Autodesk Inventor part; units mm, degrees
ref_plane "YZ Plane" through (0, 0, 0) normal (1, 0, 0) x (0, 1, 0)
ref_plane "XZ Plane" through (0, 0, 0) normal (0, 1, 0) x (-1, 0, 0)
ref_plane "XY Plane" through (0, 0, 0) normal (0, 0, 1) x (1, 0, 0)
sketch "Sketch1" plane through (0, 0, 0) normal (0, 0, 1) x (1, 0, 0)
  circle A0 centre (0, 0) radius 11.25
  circle A1 centre (0, 0) radius 12.2
  dimension "d0" = 22.5
  dimension "d1" = 24.4
extrude "Extrusion1" add sketch "Sketch1" along normal blind 6.5
sketch "Sketch2" plane through (0, 0, 0) normal (0, 0, 1) x (1, 0, 0)
  circle A0 centre (0, 0) radius 11.25
  dimension "d4" = 22.5
extrude "Extrusion2" add sketch "Sketch2" along normal blind 1
sketch "Sketch3" plane through (0, 0, 1) normal (0, 0, 1) x (1, 0, 0)
  circle A0 centre (0, 0) radius 9
  dimension "d7" = 18
extrude "Extrusion3" cut sketch "Sketch3" against normal blind 1
properties part number "HubTest22mm"
Geometry check sheet. Reference: the model listing, model coordinates, mm. A direction names the side the tool comes from. Give positions to 0.01 mm unless a question says otherwise; leave off trailing zeros. Order: outer loops, then holes, each group sorted by start corner. A loop starts at its lowest first (then second) coordinate and runs counter-clockwise, first axis right, second up.
1. Release check for a two-part mould opening along X. For faces 3 (the face through (4, -11, 6.5)), 4 (the face through (-5, 8, 1)), 5 (the face through (-12.19, -0.54, 3.2)) record: pulls with the +X half, pulls with the -X half, needs draft (parallel to the pull), parting line crosses it, or undercut.
2. Gauge pin test, flat ends, axial feed: pin 1 Ø1 at (x, z) = (-4, 5.5) entering from -Y; pin 2 Ø2 at (x, z) = (6, 4.5) entering from +Y. Record the tip position at first contact, or that the pin passes through.
3. Section check C-C, the plane z = 5.25. Enter the section's corners in (x, y), and give its area (3 significant figures).
4. Access from +Z, -Z, +X, -X, +Y, -Y to the whole of each face (thin tool, end or side, straight path). Record for faces 1 (the face through (-1.172, 8.923, 0.507)), 2 (the face through (5.19, 9.98, 3.71)).
5. Section check A-A, the plane y = 0. Enter the section's corners in (x, z).
6. Thickness scan on L1, parallel to Y at x = 0, z = 0.4; L2, parallel to Y at x = 0, z = 3; L3, parallel to X at y = -7.75, z = 4. Record the ranges inside material, lowest first.
Values follow:
1. face 3: needs draft
1. face 4: undercut
1. face 5: parting line crosses it
2. pin 1: stops at y = -11.69
2. pin 2: stops at y = 11.13
3. outline: circle Ø24.4 at (0, 0); hole circle Ø22.5 at (0, 0)
3. area: 70.0 mm2
4. face 1: +Z, -Z
4. face 2: +Z
5. outline: (-12.2, 0) - (-9, 0) - (-9, 1) - (-11.25, 1) - (-11.25, 6.5) - (-12.2, 6.5) - close; (9, 0) - (12.2, 0) - (12.2, 6.5) - (11.25, 6.5) - (11.25, 1) - (9, 1) - close
6. L1: y = -12.2 to -9, 9 to 12.2
6. L2: y = -12.2 to -11.25, 11.25 to 12.2
6. L3: x = -9.42 to -8.15, 8.15 to 9.42
